Answer from the drawing. Dimensions are ordinates in mm from the lowest x, y and z of the part. Give positions to 0.01 mm unless a question says otherwise; leave off trailing zeros. Write each loop counter-clockwise with the first axis right and the second up, starting at its lowest first coordinate (ties: lowest second). Pieces come first, ordered by that corner, then holes.
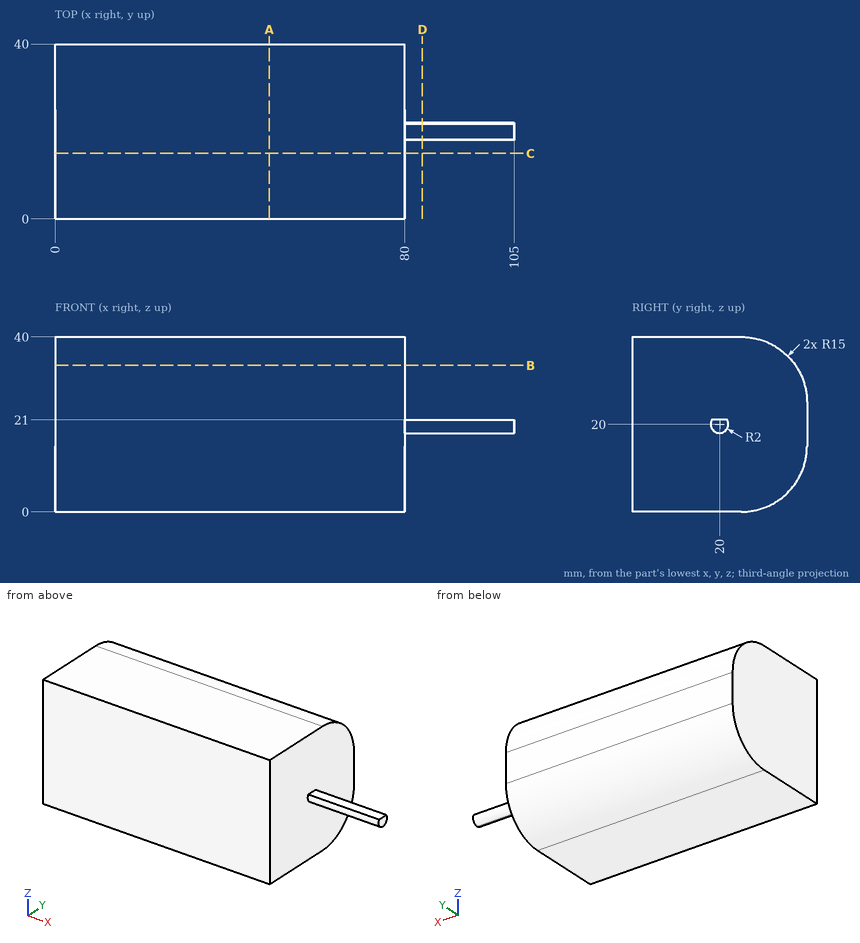
Item 1: Section D-D (x = 84) is taken. Write down the section's boundary in (y, z), and give its area (3 significant figures).
Result set:
outline: (18.27, 21) arc R2 ccw (long way) to (21.73, 21) - close
area: 10.1 mm2
Item 2: Section B-B (z = 33.5) is taken. Write down the section's boundary in (x, y).
Result set:
outline: (0, 0) - (80, 0) - (80, 37.36) - (0, 37.36) - close
Item 3: Find the intervals of material crossed by line 1 along X through (y, z) = (31, 3); line 2 along Z through (x, y) = (11, 34); line 3 along Y through (x, z) = (73.5, 3.5), in increasing order.
Result set:
line 1: x = 0 to 80
line 2: z = 3 to 37
line 3: y = 0 to 34.63
Item 4: Section A-A (x = 49) is taken. Write down the section's boundary in (y, z).
Result set:
outline: (0, 0) - (25, 0) arc R15 ccw to (40, 15) - (40, 25) arc R15 ccw to (25, 40) - (0, 40) - close
Item 5: Section C-C (y = 15) is taken. Write down the section's boundary in (x, z).
Result set:
outline: (0, 0) - (80, 0) - (80, 40) - (0, 40) - close
Item 6: Each of these flat-tipped pins is pushed along its axis until it touches: pin 1 Ø1 at (x, y) = (88.5, 19.5) entering from +Z; pin 2 Ø1 at (y, z) = (8.5, 20.5) entering from +X; pin 3 Ø1 at (x, y) = (74.5, 26) entering from -Z. Where does it stop, or does it pass through?
Result set:
pin 1: stops at z = 21
pin 2: stops at x = 80
pin 3: stops at z = 0.01
